```python
from build123d import *

# Parameters (mm, degrees)
F0_R     = 7.5
F2_DEPTH = 4
F1_W     = 37
F1_H     = 4
F3_DEPTH = 4
F5_START = -10.5
F5_DEPTH = 3
F6_W     = 29
F6_H     = 8
F7_DEPTH = 4


with BuildPart() as f2:
    # F0 (on Top) → F2 (new body)
    with BuildSketch(Plane.XY):
        Polygon((10.5, 21.05), (-10.5, 21.05), (-10.5, -21.05), (-2.25, -21.05), (-2.25, -16.55), (2.25, -16.55), (2.25, -21.05), (10.5, -21.05), align=None)
        Circle(F0_R, mode=Mode.SUBTRACT)
    extrude(amount=F2_DEPTH)

    # F1 (on Top) → F3 (join)
    with BuildSketch(Plane.XY):
        with Locations((0, 15.05)):
            Rectangle(F1_W, F1_H)
    extrude(amount=F3_DEPTH)

    # F4 (on Front) → F5 (join)
    with BuildSketch(Plane.XZ.offset(F5_START)):
        Polygon((4, -2.9999939919), (4, 0), (2, 0), (0, 0), (0, -2.9999939919), align=None)
    extrude(amount=-F5_DEPTH)

    # F6 (on Top) → F7 (join)
    with BuildSketch(Plane.XY):
        with Locations((0, 17.05)):
            Rectangle(F6_W, F6_H)
    extrude(amount=F7_DEPTH)


solid = f2.part
```
Verification items for the finished model (mm, model axes). A direction names the side the tool comes from. Coordinates: 2 decimals unless noted, no trailing zeros. Loops run counter-clockwise (first coordinate to the right, second up) from the corner with the lowest first, then second, coordinate; pieces in that order, holes last. Notation, with made-up numbers: (52.25, 8) - (110.25, 8) arc R14 ccw to (110.25, 32) - close; hole circle Ø4 at (-35, 63.5). An arc over 180 degrees is marked (long way). Answer as a JSON object with one key per item and string values.
(1) Scan lines: line 1 along X through (y, z) = (-17, 0.25); line 2 along Y through (x, z) = (0, 3.2); line 3 along Z through (x, y) = (-4, 7.5). Record each from-to range of solid material in increasing order.
Response:
{"line 1": "x = -10.5 to -2.25, 2.25 to 10.5", "line 2": "y = -16.55 to -7.5, 7.5 to 21.05", "line 3": "z = 0 to 4"}
(2) Cross-section at D-D, the plane x = 12.5. Record the boundary of the cut face in (y, z), then the cut area to 3 significant figures.
Response:
{"outline": "(13.05, 0) - (21.05, 0) - (21.05, 4) - (13.05, 4) - close", "area": "32.0 mm²"}
(3) Mould release check, pull along Y, two halves, no side actions. Record for faces 5 (the cylindrical face through (-7.493, 0.33, 1.972)), 6 (the flat face through (2, 13.5, -1)), 7 (the flat face through (0, 10, 4)): pulls with the +Y half, pulls with the -Y half, needs draft (parallel to the pull), parting line crosses it, or undercut.
Response:
{"face 5": "undercut", "face 6": "pulls with the +Y half", "face 7": "needs draft"}
(4) Access from +Z, -Z, +X, -X, +Y, -Y to the whole of each face (thin tool, end or side, straight path). Record for faces 1 (the flat face through (-17, 17.05, 2)), 2 (the flat face through (16, 17.05, 2)), 3 (the flat face through (4, 12, -2)), 4 (the flat face through (14, 13.05, 2)).
Response:
{"face 1": "+Z, -Z, -X, +Y", "face 2": "+Z, -Z, +X, +Y", "face 3": "-Z, +X, +Y, -Y", "face 4": "+Z, -Z, +X, -Y"}
(5) Go/stop test with flat-tipped pins: pin 1 Ø11 at (x, y) = (-7, -6) entering from -Z; pin 2 Ø3 at (y, z) = (0.5, 1.5) entering from +X; pin 3 Ø2 at (y, z) = (20, 2.5) entering from +X. Record where each tip stops, or that it passes through.
Response:
{"pin 1": "stops at z = 0", "pin 2": "stops at x = 10.5", "pin 3": "stops at x = 14.5"}
(6) Cross-section at B-B, the plane z = 2.5. Record the boundary of the cut face in (x, y).
Response:
{"outline": "(-18.5, 13.05) - (-10.5, 13.05) - (-10.5, -21.05) - (-2.25, -21.05) - (-2.25, -16.55) - (2.25, -16.55) - (2.25, -21.05) - (10.5, -21.05) - (10.5, 13.05) - (18.5, 13.05) - (18.5, 17.05) - (14.5, 17.05) - (14.5, 21.05) - (-14.5, 21.05) - (-14.5, 17.05) - (-18.5, 17.05) - close; hole circle Ø15 at (0, 0)"}
(7) Cross-section at C-C, the plane x = -1. Record the boundary of the cut face in (y, z).
Response:
{"outline": "(-16.55, 0) - (-7.43, 0) - (-7.43, 4) - (-16.55, 4) - close; (7.43, 0) - (21.05, 0) - (21.05, 4) - (7.43, 4) - close"}
(8) Cross-section at A-A, the plane y = 0. Record the boundary of the cut face in (x, z), then the cut area to 3 significant figures.
Response:
{"outline": "(-10.5, 0) - (-7.5, 0) - (-7.5, 4) - (-10.5, 4) - close; (7.5, 0) - (10.5, 0) - (10.5, 4) - (7.5, 4) - close", "area": "24.0 mm²"}
